```python
from build123d import *

# Parameters (mm, degrees)
SKETCH1_W                        = 25.4
SKETCH1_H                        = 25.273
BOSS_EXTRUDE1_DEPTH              = 58.42
F_54_0_055_DIAMETER_HOLE1_D      = 1.397
F_54_0_055_DIAMETER_HOLE1_DEPTH  = 12.7
F_54_0_055_DIAMETER_HOLE1_TIP    = 0.419701142
F_3_8_0_375_DIAMETER_HOLE2_D     = 9.525
F_3_8_0_375_DIAMETER_HOLE2_DEPTH = 50.8
F_3_8_0_375_DIAMETER_HOLE2_TIP   = 2.861598698
F_10_32_TAPPED_HOLE1_D           = 4.0386
F_10_32_TAPPED_HOLE1_DEPTH       = 8.946682152
F_10_32_TAPPED_HOLE1_TIP         = 1.213317848


with BuildPart() as part:
    # Sketch1 → Boss-Extrude1 (new body)
    with BuildSketch(Plane(origin=(0, 0, 0), x_dir=(1, 0, 0), z_dir=(0, 1, 0))):
        with Locations((-12.7, 12.6365)):
            Rectangle(SKETCH1_W, SKETCH1_H)
    extrude(amount=BOSS_EXTRUDE1_DEPTH)

    # #54 (0.055) Diameter Hole1
    with Locations(Plane(origin=(-12.7, 7.62, 0), x_dir=(1, 0, 0), z_dir=(0, 0, 1))):
        with Locations((0, 0)):
            Hole(F_54_0_055_DIAMETER_HOLE1_D / 2, depth=F_54_0_055_DIAMETER_HOLE1_DEPTH)
            with Locations((0, 0, -(F_54_0_055_DIAMETER_HOLE1_DEPTH + F_54_0_055_DIAMETER_HOLE1_TIP / 2))):  # 118° drill point
                Cone(0, F_54_0_055_DIAMETER_HOLE1_D / 2, F_54_0_055_DIAMETER_HOLE1_TIP, mode=Mode.SUBTRACT)

    # 3/8 (0.375) Diameter Hole2
    with Locations(Plane(origin=(-12.7, 58.42, -16.002), x_dir=(0, 0, 1), z_dir=(0, 1, 0))):
        with Locations((0, 0)):
            Hole(F_3_8_0_375_DIAMETER_HOLE2_D / 2, depth=F_3_8_0_375_DIAMETER_HOLE2_DEPTH)
            with Locations((0, 0, -(F_3_8_0_375_DIAMETER_HOLE2_DEPTH + F_3_8_0_375_DIAMETER_HOLE2_TIP / 2))):  # 118° drill point
                Cone(0, F_3_8_0_375_DIAMETER_HOLE2_D / 2, F_3_8_0_375_DIAMETER_HOLE2_TIP, mode=Mode.SUBTRACT)

    # #10-32 Tapped Hole1
    with Locations(Plane(origin=(-12.7, 26.67, 0), x_dir=(1, 0, 0), z_dir=(0, 0, 1))):
        with Locations((0, 0)):
            Hole(F_10_32_TAPPED_HOLE1_D / 2, depth=F_10_32_TAPPED_HOLE1_DEPTH)
            with Locations((0, 0, -(F_10_32_TAPPED_HOLE1_DEPTH + F_10_32_TAPPED_HOLE1_TIP / 2))):  # 118° drill point
                Cone(0, F_10_32_TAPPED_HOLE1_D / 2, F_10_32_TAPPED_HOLE1_TIP, mode=Mode.SUBTRACT)


solid = part.part
```
The model under review builds one solid part; all positions refer to its coordinate system, in mm. A direction names the side the tool comes from. Give positions to 0.01 mm unless a question says otherwise; leave off trailing zeros. Loops run counter-clockwise (first coordinate to the right, second up) from the corner with the lowest first, then second, coordinate; pieces in that order, holes last. Notation, with made-up numbers: (88, 7) -> (126, 7) arc R22 ccw to (126, 26) -> close; hole circle Ø10 at (1.5, -38.5). An arc over 180 degrees is marked (long way). Use CSV: the item, a comma, the result in double quotes.
1. The part is to be moulded in two halves that separate along Z. For faces 1 (the face through (-13.434, 5.255, -15.62)), 2 (the face through (-13, 29, 0)), 3 (the face through (-12.549, 6.938, -6.288)), say which applies: +Z half, -Z half, draft (parallel to the pull), parting line (faces both ways), or undercut.
Result:
face 1,"undercut"
face 2,"+Z half"
face 3,"draft"
2. To check wall thickness, follow probe 1 along Y at (x, z) = (-12.7, -8.5); probe 2 along X at (y, z) = (26.67, -5.25); probe 3 along X at (y, z) = (53.5, -16). State the ranges of each line that lie inside material, in increasing order. Write a range as from..to.
Result:
probe 1,"y = 0..6.92, 8.32..24.65, 28.69..58.42"
probe 2,"x = -25.4..-14.72, -10.68..0"
probe 3,"x = -25.4..-17.46, -7.94..0"
3. Consider section A-A, the plane y = 50.5. Write out the cut boundary in (x, z) (1 decimal), then the cut area to 3 significant figures.
Result:
outline,"(-25.4, -25.3) -> (0, -25.3) -> (0, 0) -> (-25.4, 0) -> close; hole circle Ø9.5 at (-12.7, -16)"
area,"571 mm²"
4. Machinability: for faces 4 (the face through (-11.21, 28.03, -4.54)), 5 (the face through (-12.491, 32.664, -11.244)), 6 (the face through (-13, 29, -25.273)), which of the approach directions +Z, -Z, +X, -X, +Y, -Y give a long, thin tool a straight path to every point of the face, cutting with its end or side? Answer none if there is none.
Result:
face 4,"+Z"
face 5,"+Y"
face 6,"-Z, +X, -X, +Y, -Y"
5. For P1, Ø2, axis at x = -10.5, y = 34.5, coming from the +Z side, flat-tipped, find the tip position at first contact; note if it passes through.
Result:
P1,"stops at z = 0"
